CAD build for the part. Positions are in the model's coordinates, mm. Coordinates: 2 decimals unless noted, no trailing zeros. Answer as CSV lines item,"result". Start each with the question number.
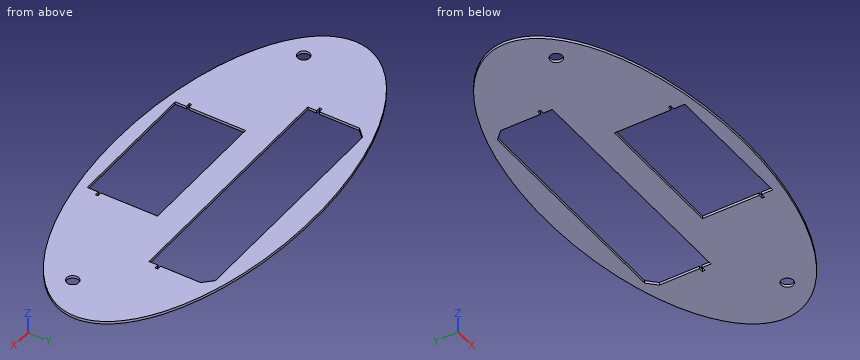
from build123d import *

# Parameters (mm, degrees)
SKETCH1_RX          = 244
SKETCH1_RY          = 110
BOSS_EXTRUDE1_DEPTH = 3
CUT_EXTRUDE5_DEPTH  = 4
CUT_EXTRUDE7_DEPTH  = 4
SKETCH12_R          = 6.83635542
CUT_EXTRUDE8_DEPTH  = 4
CHAMFER1_SIZE       = 10


with BuildPart() as part:
    # Sketch1 → Boss-Extrude1 (new body)
    with BuildSketch(Plane.XY):
        with Locations((0, 0)):
            Ellipse(SKETCH1_RX, SKETCH1_RY)
    extrude(amount=-BOSS_EXTRUDE1_DEPTH)

    # Sketch10 → Cut-Extrude5 (cut, through all)
    with BuildSketch(Plane.XY):
        Polygon((-137.5, 83.1), (137.5, 83.1), (137.5, 28.1), (142.5, 28.1), (142.5, 25.1), (137.5, 25.1), (137.5, 15.1), (-137.5, 15.1), (-137.5, 25.1), (-142.5, 25.1), (-142.5, 28.1), (-137.5, 28.1), align=None)
    extrude(amount=-CUT_EXTRUDE5_DEPTH, mode=Mode.SUBTRACT)

    # Sketch13 → Cut-Extrude7 (cut, through all)
    with BuildSketch(Plane.XY):
        Polygon((76.2, -81.5), (76.2, -93.9), (-76.2, -93.9), (-76.2, -81.5), (-81.2, -81.5), (-81.2, -78.5), (-76.2, -78.5), (-76.2, -15), (76.2, -15), (76.2, -78.5), (81.2, -78.5), (81.2, -81.5), align=None)
    extrude(amount=-CUT_EXTRUDE7_DEPTH, mode=Mode.SUBTRACT)

    # Sketch12 → Cut-Extrude8 (cut, through all)
    with BuildSketch(Plane.XY):
        with Locations((200, -30)):
            Circle(SKETCH12_R)
        with Locations((-200, -30)):
            Circle(SKETCH12_R)
    extrude(amount=-CUT_EXTRUDE8_DEPTH, mode=Mode.SUBTRACT)

    # Chamfer1
    chamfer1_edges = [part.edges().sort_by_distance(p)[0] for p in [
        (-137.5, 83.1, -1.5),
        (137.5, 83.1, -1.5),
    ]]
    chamfer(chamfer1_edges, length=CHAMFER1_SIZE)


solid = part.part
Item 1: Flat gauge pins, fed straight in: pin 1 Ø1 at (y, z) = (-76.5, -0.5) entering from -X; pin 2 Ø0.9 at (x, z) = (-15, -1) entering from -Y; pin 3 Ø0.9 at (x, z) = (80, -1.5) entering from -Y. Where does each tip first touch, or does it go through?
Item 2: Wall check: probe 1 along Y at (x, z) = (50, -2.5); probe 2 along X at (y, z) = (28, -2.6); probe 3 along Y at (x, z) = (-200, -1.1). Give the ranges that are in metal, low to high.
Item 3: Saw through at A-A (x = -40). Count the separate pieces of the cut face and the enclosed holes in it, plus the area to 3 significant figures.
Geometry check:
1,pin 1,"x = -176.4"
1,pin 2,"y = -109.8"
1,pin 3,"y = -103.99"
2,probe 1,"-107.67 to -93.9, -15 to 15.1, 83.1 to 107.67"
2,probe 2,"-235.96 to -142.5, 142.5 to 235.96"
2,probe 3,"-63.01 to -36.84, -23.16 to 63.01"
3,separate pieces,"3"
3,enclosed holes,"0"
3,area,"210 mm2"
